from build123d import *

# Parameters (mm, degrees)
SKETCH1_W           = 40
SKETCH1_H           = 50
BOSS_EXTRUDE2_DEPTH = 15
SKETCH2_W           = 34
SKETCH2_H           = 7
CUT_EXTRUDE1_DEPTH  = 50
SKETCH3_W           = 7
SKETCH3_H           = 30
CUT_EXTRUDE2_DEPTH  = 50
SKETCH6_W           = 40
SKETCH6_H           = 2.5
SKETCH6_H_2         = 4.98530806
CUT_EXTRUDE4_DEPTH  = 50
SKETCH7_W           = 40
SKETCH7_H           = 12.5
CUT_EXTRUDE5_DEPTH  = 5
SKETCH8_W           = 20
SKETCH8_H           = 12.51469194
CUT_EXTRUDE7_DEPTH  = 5
SKETCH11_R          = 2.5
CUT_EXTRUDE10_DEPTH = 5
SKETCH12_R          = 1.5
CUT_EXTRUDE11_DEPTH = 15
FILLET2_R           = 5
FILLET3_R           = 5


with BuildPart() as part:
    # Sketch1 → Boss-Extrude2 (new body)
    with BuildSketch(Plane.XY):
        with Locations((400.458722726, 329.091279026)):
            Rectangle(SKETCH1_W, SKETCH1_H)
    extrude(amount=BOSS_EXTRUDE2_DEPTH)

    # Sketch2 → Cut-Extrude1 (cut)
    with BuildSketch(Plane(origin=(0, 354.091279026, 0), x_dir=(1, 0, 0), z_dir=(0, 1, 0))):
        with Locations((400.458722726, -8.5)):
            Rectangle(SKETCH2_W, SKETCH2_H)
    extrude(amount=-CUT_EXTRUDE1_DEPTH, mode=Mode.SUBTRACT)

    # Sketch3 → Cut-Extrude2 (cut)
    with BuildSketch(Plane.ZY.offset(-380.458722726)):
        with Locations((8.5, 339.091279026)):
            Rectangle(SKETCH3_W, SKETCH3_H)
    extrude(amount=-CUT_EXTRUDE2_DEPTH, mode=Mode.SUBTRACT)

    # Sketch6 → Cut-Extrude4 (cut)
    with BuildSketch(Plane(origin=(0, 0, 0), x_dir=(-1, 0, 0), z_dir=(0, 0, -1))):
        with Locations((-400.458722726, 352.841279026)):
            Rectangle(SKETCH6_W, SKETCH6_H)
        with Locations((-400.458722726, 306.583933056)):
            Rectangle(SKETCH6_W, SKETCH6_H_2)
    extrude(amount=-CUT_EXTRUDE4_DEPTH, mode=Mode.SUBTRACT)

    # Sketch7 → Cut-Extrude5 (cut)
    with BuildSketch(Plane.XY.offset(15)):
        with Locations((400.458722726, 345.341279026)):
            Rectangle(SKETCH7_W, SKETCH7_H)
    extrude(amount=-CUT_EXTRUDE5_DEPTH, mode=Mode.SUBTRACT)

    # Sketch8 → Cut-Extrude7 (cut)
    with BuildSketch(Plane.XY.offset(15)):
        with Locations((400.458722726, 322.833933056)):
            Rectangle(SKETCH8_W, SKETCH8_H)
    extrude(amount=-CUT_EXTRUDE7_DEPTH, mode=Mode.SUBTRACT)

    # Sketch11 → Cut-Extrude10 (cut)
    with BuildSketch(Plane.XY.offset(5)):
        with Locations((400.458722726, 344.660615353)):
            Circle(SKETCH11_R)
        with Locations((400.458722726, 322.932953385)):
            Circle(SKETCH11_R)
    extrude(amount=-CUT_EXTRUDE10_DEPTH, mode=Mode.SUBTRACT)

    # Sketch12 → Cut-Extrude11 (cut)
    with BuildSketch(Plane.XY.offset(15)):
        with Locations((415.958722726, 334.091279026)):
            Circle(SKETCH12_R)
        with Locations((384.958722726, 334.091279026)):
            Circle(SKETCH12_R)
    extrude(amount=-CUT_EXTRUDE11_DEPTH, mode=Mode.SUBTRACT)

    # Fillet2
    fillet2_edges = [part.edges().sort_by_distance(p)[0] for p in [
        (380.458722726, 339.091279026, 13.5),
    ]]
    fillet(fillet2_edges, radius=FILLET2_R)

    # Fillet3
    fillet3_edges = [part.edges().sort_by_distance(p)[0] for p in [
        (420.458722726, 339.091279026, 13.5),
        (380.458722726, 351.591279026, 2.5),
        (420.458722726, 351.591279026, 2.5),
    ]]
    fillet(fillet3_edges, radius=FILLET3_R)


solid = part.part
Geometry: final body of the model. Coordinates: model frame, mm. A direction names the side the tool comes from. Round coordinates to 2 decimals unless told otherwise and drop trailing zeros. Order: outer loops, then holes, each group sorted by start corner. A loop starts at its lowest first (then second) coordinate and runs counter-clockwise, first axis right, second up. Notation, with made-up numbers: (76, 37.25) - (120, 37.25) arc R11 cw to (120, 49.25) - close; hole circle Ø9 at (73, 71.5). An arc over 180 degrees is marked (long way). Write each question's results on one line, items separated by ' | '.
Item 1: Mould query, pull axis X, two halves, no side actions, for faces 6 (the cylindrical face through (418.955, 350.165, 2.535)), 7 (the cylindrical face through (416.765, 335.356, 2.535)), 8 (the flat face through (401, 351.591, 2)). Classes: pulls with the +X half, pulls with the -X half, needs draft (parallel to the pull), parting line crosses it, or undercut.
Completed:
face 6: pulls with the +X half | face 7: undercut | face 8: needs draft
Item 2: First-contact query: pin 1 Ø2.5 at (x, z) = (398.5, 14) entering from +Y; pin 2 Ø3.5 at (x, y) = (384.96, 334.09) entering from -Z; pin 3 Ø1.8 at (x, y) = (384.96, 334.09) entering from -Z; pin 4 Ø3.5 at (x, z) = (382, 10) entering from +Y. Flat tips, straight axial feed; report the tip coordinate or a pass-through.
Completed:
pin 1: y = 339.09 | pin 2: z = 0 | pin 3: through | pin 4: y = 324.09
Item 3: Section D-D, the plane y = 332. Return the cut outline in (x, z).
Completed:
outline: (380.46, 0) - (420.46, 0) - (420.46, 5) - (380.46, 5) - close; (380.46, 12) - (420.46, 12) - (420.46, 15) - (380.46, 15) - close
Item 4: Section B-B, the plane x = 404. Return the cut outline in (y, z), and give its area (3 significant figures).
Completed:
outline: (309.08, 0) - (351.59, 0) - (351.59, 5) - (309.08, 5) - close; (309.08, 12) - (316.58, 12) - (316.58, 15) - (309.08, 15) - close; (329.09, 12) - (339.09, 12) - (339.09, 15) - (329.09, 15) - close | area: 265 mm^2
Item 5: Reachability of faces 1 (the flat face through (400, 339.091, 14)), 2 (the flat face through (410.459, 323, 14)), 3 (the cylindrical face through (418.955, 337.665, 13.479)), 4 (the flat face through (382, 324.091, 8)), 5 (the flat face through (417.459, 317, 9)) from +Z, -Z, +X, -X, +Y, -Y: full face, straight path, thin tool, end or side. Return the list, or none.
Completed:
face 1: +Z, +X, -X, +Y | face 2: +Z | face 3: +Z, +X, +Y | face 4: +X, -X, +Y | face 5: +Y, -Y
Item 6: Section C-C, the plane z = 14. Return the cut outline in (x, y), and give its area (3 significant figures).
Completed:
outline: (380.46, 309.08) - (420.46, 309.08) - (420.46, 334.09) arc R5 ccw to (415.46, 339.09) - (385.46, 339.09) arc R5 ccw to (380.46, 334.09) - close; hole circle Ø3 at (384.96, 334.09); hole (390.46, 316.58) - (410.46, 316.58) - (410.46, 329.09) - (390.46, 329.09) - close; hole circle Ø3 at (415.96, 334.09) | area: 925 mm^2
Item 7: Section A-A, the plane x = 411.5. Return the cut outline in (y, z), and give its area (3 significant figures).
Completed:
outline: (309.08, 0) - (351.59, 0) - (351.59, 5) - (309.08, 5) - close; (309.08, 12) - (339.09, 12) - (339.09, 15) - (309.08, 15) - close | area: 303 mm^2
Item 8: Material intervals for line 1 along Z through (x, y) = (397.5, 338.5); line 2 along Y through (x, z) = (395, 13); line 3 along Z through (x, y) = (399.5, 326.5), sorted ascending. Write a range as [from, to].
Completed:
line 1: [0, 5], [12, 15] | line 2: [309.08, 316.58], [329.09, 339.09] | line 3: [0, 5]
